Work out the finished part from the listing and answer in its coordinate system (mm). Face numbers are marked on the shaded views. A direction names the side the tool comes from. Coordinates: 2 decimals unless noted, no trailing zeros. Order: outer loops, then holes, each group sorted by start corner. A loop starts at its lowest first (then second) coordinate and runs counter-clockwise, first axis right, second up. Notation, with made-up numbers: M -8,36.25 L 15,36.25 A28 ccw 15,56.25 Z; hole C 35.5,-27 d6. An arc over 180 degrees is marked long. Use a Markdown table: item, result.
from build123d import *

# Parameters (mm, degrees)
F0_W      = 70
F0_H      = 70
F0_R      = 20
F3_DEPTH  = 50
F4_D      = 10
F4_DEPTH  = 45
F4_TIP    = 3.0043030951
F5_D      = 10
F5_DEPTH  = 45
F5_TIP    = 3.0043030951
F7_R      = 5
F8_R      = 5
F9_R      = 5
F10_R     = 5
F11_D     = 60
F11_DEPTH = 45
F11_TIP   = 18.0258185708


with BuildPart() as f3:
    # F0 (on Top) → F3 (new body)
    with BuildSketch(Plane.XY):
        with Locations((-35, 35)):
            Rectangle(F0_W, F0_H)
        with Locations((-35, 35)):
            Circle(F0_R, mode=Mode.SUBTRACT)
    extrude(amount=F3_DEPTH)

    # F4
    with Locations(Plane(origin=(0, 0, 0), x_dir=(1, 0, 0), z_dir=(0, 0, -1))):
        with Locations((-64, -17)):
            Hole(F4_D / 2, depth=F4_DEPTH)
            with Locations((0, 0, -(F4_DEPTH + F4_TIP / 2))):  # 118° drill point
                Cone(0, F4_D / 2, F4_TIP, mode=Mode.SUBTRACT)

    # F5
    with Locations(Plane(origin=(0, 0, 0), x_dir=(1, 0, 0), z_dir=(0, 0, -1))):
        with Locations((-6, -53), (-6, -17), (-64, -53)):
            Hole(F5_D / 2, depth=F5_DEPTH)
            with Locations((0, 0, -(F5_DEPTH + F5_TIP / 2))):  # 118° drill point
                Cone(0, F5_D / 2, F5_TIP, mode=Mode.SUBTRACT)

    # F7
    f7_edges = [f3.edges().sort_by_distance(p)[0] for p in [
        (0, 0, 25),
    ]]
    fillet(f7_edges, radius=F7_R)

    # F8
    f8_edges = [f3.edges().sort_by_distance(p)[0] for p in [
        (-70, 0, 25),
    ]]
    fillet(f8_edges, radius=F8_R)

    # F9
    f9_edges = [f3.edges().sort_by_distance(p)[0] for p in [
        (0, 70, 25),
    ]]
    fillet(f9_edges, radius=F9_R)

    # F10
    f10_edges = [f3.edges().sort_by_distance(p)[0] for p in [
        (-70, 70, 25),
    ]]
    fillet(f10_edges, radius=F10_R)

    # F11
    with Locations(Plane(origin=(0, 0, 0), x_dir=(1, 0, 0), z_dir=(0, 0, -1))):
        with Locations((-35, -35)):
            Hole(F11_D / 2, depth=F11_DEPTH)
            with Locations((0, 0, -(F11_DEPTH + F11_TIP / 2))):  # 118° drill point
                Cone(0, F11_D / 2, F11_TIP, mode=Mode.SUBTRACT)


solid = f3.part
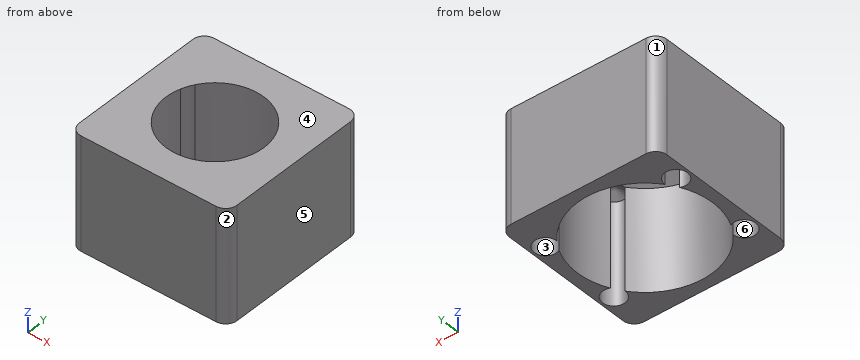
(1) Which of the six approach directions +Z, -Z, +X, -X, +Y, -Y give full straight-line access (tool end or side, diameter ignored) to the marked faces 5 and 6?
Conclusion:
| item | result |
|---|---|
| face 5 | +Z, -Z, +X, +Y, -Y |
| face 6 | -Z |
(2) A cutting plane is placed at B-B (y = 35). Determine the outline of the cut face in (x, z), then the cut area to 3 significant figures.
Conclusion:
| item | result |
|---|---|
| outline | M -70,0 L -65,0 L -65,45 L -56.68,50 L -70,50 Z; M -13.32,50 L -5,45 L -5,0 L 0,0 L 0,50 Z |
| area | 542 mm2 |
(3) Straight lines are drawn through the part: L1, parallel to Y at x = -3, z = 23; L2, parallel to X at y = 54, z = 7; L3, parallel to Y at x = -12.5, z = 20.5. For each, find the intervals that lie inside material, in ascending order.
Conclusion:
| item | result |
|---|---|
| L1 | 0.42 to 13, 21 to 49, 57 to 69.58 |
| L2 | -70 to -68.9, -59.1 to -58.22, -11.78 to -10.9, -1.1 to 0 |
| L3 | 0 to 15.16, 54.84 to 70 |
(4) A cutting plane is placed at A-A (z = 22). Determine the outline of the cut face in (x, y), then the cut area to 3 significant figures.
Conclusion:
| item | result |
|---|---|
| outline | M -70,5 A5 ccw -65,0 L -5,0 A5 ccw 0,5 L 0,65 A5 ccw -5,70 L -65,70 A5 ccw -70,65 Z; hole M -61.78,21.48 A5 ccw long -59,17 A30 ccw -11,17 A5 ccw long -8.22,21.48 A30 ccw -8.22,48.52 A5 ccw long -11,53 A30 ccw -59,53 A5 ccw long -61.78,48.52 A30 ccw Z |
| area | 1,750 mm2 |
(5) Given P1, Ø1, axis at x = -10.5, y = 36, coming from the -Z side; P2, Ø4, axis at x = -41, y = 9.5, coming from the -Z side, each flat-ended and moving along its own axis, determine where each tip first touches the part or whether it passes through.
Conclusion:
| item | result |
|---|---|
| P1 | z = 47.99 |
| P2 | z = 46.08 |
(6) Determine the mould class of the marked faces 1, 2, 3 and 4 for opening direction Y: pulls with the +Y half, pulls with the -Y half, needs draft (parallel to the pull), parting line crosses it, or undercut.
Conclusion:
| item | result |
|---|---|
| face 1 | pulls with the +Y half |
| face 2 | pulls with the -Y half |
| face 3 | undercut |
| face 4 | needs draft |
